```python
from build123d import *

# Parameters (mm, degrees)
SKIZZE1_W                            = 160
SKIZZE1_H                            = 300
SKIZZE1_W_2                          = 100
SKIZZE1_H_2                          = 27
AUFSATZ_LINEAR_AUSTRAGEN1_DEPTH      = 20
SKIZZE2_W                            = 100
SKIZZE2_H                            = 20
AUFSATZ_LINEAR_AUSTRAGEN2_DEPTH      = 90
AUFSATZ_LINEAR_AUSTRAGEN2_DEPTH_BACK = 20
M6_GEWINDEBOHRUNG1_D                 = 5
M6_GEWINDEBOHRUNG1_CSINK_D           = 6.05
M6_GEWINDEBOHRUNG1_CSINK_ANGLE       = 90


with BuildPart() as part:
    # Skizze1 → Aufsatz-Linear austragen1 (new body)
    with BuildSketch(Plane.XY):
        with Locations((80, 150)):
            Rectangle(SKIZZE1_W, SKIZZE1_H)
        Polygon((0, 0), (160, 0), (130, -33), (30, -33), align=None)
        with Locations((80, -46.5)):
            Rectangle(SKIZZE1_W_2, SKIZZE1_H_2)
    extrude(amount=AUFSATZ_LINEAR_AUSTRAGEN1_DEPTH)

    # Skizze2 → Aufsatz-Linear austragen2 (add, two sides)
    with BuildSketch(Plane.XY.offset(20)) as aufsatz_linear_austragen2_sk:
        with Locations((80, -70)):
            Rectangle(SKIZZE2_W, SKIZZE2_H)
    extrude(amount=AUFSATZ_LINEAR_AUSTRAGEN2_DEPTH)
    extrude(aufsatz_linear_austragen2_sk.sketch, amount=-AUFSATZ_LINEAR_AUSTRAGEN2_DEPTH_BACK)

    # M6 Gewindebohrung1 (through all)
    with Locations(Plane(origin=(0, -60, 0), x_dir=(1, 0, 0), z_dir=(0, 1, 0))):
        with Locations((50, -97.5), (110, -97.5), (110, -42.5), (50, -42.5)):
            CounterSinkHole(M6_GEWINDEBOHRUNG1_D / 2, M6_GEWINDEBOHRUNG1_CSINK_D / 2, counter_sink_angle=M6_GEWINDEBOHRUNG1_CSINK_ANGLE)


solid = part.part
```
Check sheet for the modelled part. Datum: model origin and axes. Units: mm. A direction names the side the tool comes from. Give positions to 0.01 mm unless a question says otherwise; leave off trailing zeros. Write each loop counter-clockwise with the first axis right and the second up, starting at its lowest first coordinate (ties: lowest second). Pieces come first, ordered by that corner, then holes.
Item 1: Scan lines: L1, parallel to Z at x = 50, y = -70; L2, parallel to X at y = -65.75, z = 97.5; L3, parallel to X at y = -76, z = 42. Record each from-to range of solid material in increasing order.
Item 2: Gauge pin test, flat ends, axial feed: pin 1 (4 mm diameter, centred on x = 52, y = -3, fed in from +Z); pin 2 (3 mm diameter, centred on x = 93, z = 93, fed in from +Y). Record the tip position at first contact, or that the pin passes through.
Item 3: Draft check along Z on faces 1 (the face through (79, -70, 110)), 2 (the face through (130, -67, 44)), 3 (the face through (79, 113, 0)). Enter one of: released by +Z, released by -Z, zero draft, split by the parting line, or undercut.
Item 4: Access from +Z, -Z, +X, -X, +Y, -Y to the whole of each face (thin tool, end or side, straight path). Record for faces 4 (the face through (30, -67, 44)), 5 (the face through (79, -60, 64)), 6 (the face through (145.21, -16.27, 9.86)).
Item 5: Cross-section at A-A (z = 12). Enter the section's corners in (x, y), and give its area (3 significant figures).
Item 6: Cross-section at B-B (x = 58). Enter the section's corners in (y, z), and give its area (3 significant figures).
Item 7: Cross-section at C-C (y = 50.5). Enter the section's corners in (x, z).
Item 8: Cross-section at D-D (x = 133.5). Enter the section's corners in (y, z), and give its area (3 significant figures).
Report:
1. L1: z = 0 to 40, 45 to 95, 100 to 110
1. L2: x = 30 to 47.5, 52.5 to 107.5, 112.5 to 130
1. L3: x = 30 to 47.55, 52.45 to 107.55, 112.45 to 130
2. pin 1: stops at z = 20
2. pin 2: stops at y = -60
3. face 1: released by +Z
3. face 2: zero draft
3. face 3: released by -Z
4. face 4: +Z, -Z, -X, -Y
4. face 5: +Z, +X, -X, +Y
4. face 6: +Z, -Z, +X, -Y
5. outline: (0, 0) - (30, -33) - (30, -80) - (130, -80) - (130, -33) - (160, 0) - (160, 300) - (0, 300) - close
5. area: 57,000 mm2
6. outline: (-80, 0) - (300, 0) - (300, 20) - (-60, 20) - (-60, 110) - (-80, 110) - close
6. area: 9,400 mm2
7. outline: (0, 0) - (160, 0) - (160, 20) - (0, 20) - close
8. outline: (-29.15, 0) - (300, 0) - (300, 20) - (-29.15, 20) - close
8. area: 6,580 mm2
